```python
from build123d import *

# Parameters (mm, degrees)
SKETCH1_R           = 0.5
BOSS_EXTRUDE1_DEPTH = 3
SKETCH2_W           = 20
SKETCH2_H           = 3
BOSS_EXTRUDE2_DEPTH = 6


with BuildPart() as part:
    # Sketch1 → Boss-Extrude1 (new body)
    with BuildSketch(Plane.XY):
        Polygon((0, 0), (9, 0), (9, 3), (14.5, 3), (14.5, 9), (-5.5, 9), (-5.5, 3), (0, 3), align=None)
        with Locations((4.5, 6)):
            Circle(SKETCH1_R, mode=Mode.SUBTRACT)
    extrude(amount=BOSS_EXTRUDE1_DEPTH)

    # Sketch2 → Boss-Extrude2 (add)
    with BuildSketch(Plane.XZ):
        with Locations((4.5, 1.5)):
            Rectangle(SKETCH2_W, SKETCH2_H)
    extrude(amount=BOSS_EXTRUDE2_DEPTH)


solid = part.part
```
Check sheet for the modelled part. Datum: model origin and axes. Units: mm. A direction names the side the tool comes from. Coordinates: 2 decimals unless noted, no trailing zeros. Loops run counter-clockwise (first coordinate to the right, second up) from the corner with the lowest first, then second, coordinate; pieces in that order, holes last.
1) Sectioned sample at B-B (x = 4.5). Record the boundary of the cut face in (y, z).
2) Material ranges on probe 1 along Y at (x, z) = (-1, 0.9); probe 2 along Y at (x, z) = (4.5, 2); probe 3 along X at (y, z) = (1, 0.4), recorded low to high.
3) Sectioned sample at A-A (y = 6). Record the boundary of the cut face in (x, z), and give its area (3 significant figures).
4) Sectioned sample at D-D (y = 2.5). Record the boundary of the cut face in (x, z).
5) Gauge pin test, flat ends, axial feed: pin 1 (8 mm diameter, centred on x = -2.5, y = 2, fed in from -Z); pin 2 (0.9 mm diameter, centred on y = 2, z = 1, fed in from +X). Record the tip position at first contact, or that the pin passes through.
6) Access from +Z, -Z, +X, -X, +Y, -Y to the whole of each face (thin tool, end or side, straight path). Record for faces 1 (the face through (9, 1, 1)), 2 (the face through (4, 2, 3)), 3 (the face through (-3, 3, 1)).
7) Release check for a two-part mould opening along Y. For faces 4 (the face through (14.5, -3, 1)), 5 (the face through (12, 0, 2)), 6 (the face through (5, 9, 1)) record: released by +Y, released by -Y, zero draft, split by the parting line, or undercut.
8) Sectioned sample at C-C (z = 1.6). Record the boundary of the cut face in (x, y).
Check sheet entries:
1. outline: (-6, 0) - (5.5, 0) - (5.5, 3) - (-6, 3) - close; (6.5, 0) - (9, 0) - (9, 3) - (6.5, 3) - close
2. probe 1: y = -6 to 0, 3 to 9
2. probe 2: y = -6 to 5.5, 6.5 to 9
2. probe 3: x = 0 to 9
3. outline: (-5.5, 0) - (4, 0) - (4, 3) - (-5.5, 3) - close; (5, 0) - (14.5, 0) - (14.5, 3) - (5, 3) - close
3. area: 57.0 mm2
4. outline: (0, 0) - (9, 0) - (9, 3) - (0, 3) - close
5. pin 1: stops at z = 0
5. pin 2: stops at x = 9
6. face 1: +Z, -Z, +X
6. face 2: +Z, +X, -X, +Y, -Y
6. face 3: +Z, -Z, -X
7. face 4: zero draft
7. face 5: undercut
7. face 6: released by +Y
8. outline: (-5.5, -6) - (14.5, -6) - (14.5, 0) - (9, 0) - (9, 3) - (14.5, 3) - (14.5, 9) - (-5.5, 9) - (-5.5, 3) - (0, 3) - (0, 0) - (-5.5, 0) - close; hole circle Ø1 at (4.5, 6)
